The listing builds one solid part. Answer for the finished solid, in the listing's coordinates (mm). A direction names the side the tool comes from. Coordinates: 2 decimals unless noted, no trailing zeros. Order: outer loops, then holes, each group sorted by start corner. A loop starts at its lowest first (then second) coordinate and runs counter-clockwise, first axis right, second up. Notation, with made-up numbers: (-37, -8) -> (-11, -8) arc R22 ccw to (-11, 25) -> close; hole circle Ø11 at (20.5, -3.75). An arc over 180 degrees is marked (long way). Answer in a Markdown table with one row per item.
```python
from build123d import *

# Parameters (mm, degrees)
BOSS_EXTRUDE1_DEPTH          = 4
SKETCH3_R                    = 1.5
BOSS_EXTRUDE2_DEPTH          = 6
F_3_0_3_DIAMETER_HOLE1_D     = 3
F_3_0_3_DIAMETER_HOLE1_DEPTH = 10
FILLET2_R                    = 14.5
FILLET3_R                    = 2
CUT_EXTRUDE1_DEPTH           = 74.871510978
CUT_EXTRUDE1_DEPTH_BACK      = 7
SKETCH8_R                    = 46
SKETCH8_R_2                  = 9.814954576


with BuildPart() as part:
    # Sketch1 → Revolve1 (revolve)
    with BuildSketch(Plane(origin=(0, 0, 0), x_dir=(1, 0, 0), z_dir=(0, 1, 0))):
        Polygon((28, 45.5), (0, 45.5), (0, 16.5), (36, 16.5), (46, 26.5), (46, 40.5), align=None)
    revolve(axis=Axis((0, 0, -45.5), (0, 0, 1)))

    # Sketch2 → Boss-Extrude1 (add)
    with BuildSketch(Plane(origin=(0, 0, -45.5), x_dir=(-1, 0, 0), z_dir=(0, 0, -1))):
        Polygon((-9.814954576, 0), (-4.907477288, 8.5), (4.907477288, 8.5), (9.814954576, 0), (4.907477288, -8.5), (-4.907477288, -8.5), align=None)
    extrude(amount=BOSS_EXTRUDE1_DEPTH)

    # Sketch3 → Boss-Extrude2 (add)
    with BuildSketch(Plane.XY.offset(-16.5)):
        Circle(SKETCH3_R)
    extrude(amount=BOSS_EXTRUDE2_DEPTH)

    # Ø3.0 (3) Diameter Hole1
    with Locations(Plane.XY.offset(-16.5)):
        with Locations((-15.5, 0), (0, 15.5), (0, -15.5), (15.5, 0)):
            Hole(F_3_0_3_DIAMETER_HOLE1_D / 2, depth=F_3_0_3_DIAMETER_HOLE1_DEPTH)

    # Fillet2
    fillet2_edges = [part.edges().sort_by_distance(p)[0] for p in [
        (-36, 0, -16.5),
    ]]
    fillet(fillet2_edges, radius=FILLET2_R)

    # Fillet3
    fillet3_edges = [part.edges().sort_by_distance(p)[0] for p in [
        (-46, 0, -26.5),
    ]]
    fillet(fillet3_edges, radius=FILLET3_R)

    # Sketch8 → Cut-Extrude1 (cut, two sides: drawn at the far end of the back side and taken through both)
    with BuildSketch(Plane(origin=(0, 0, -45.5), x_dir=(-1, 0, 0), z_dir=(0, 0, -1)).offset(-CUT_EXTRUDE1_DEPTH_BACK)):
        Circle(SKETCH8_R)
        Circle(SKETCH8_R_2, mode=Mode.SUBTRACT)
    extrude(amount=CUT_EXTRUDE1_DEPTH + CUT_EXTRUDE1_DEPTH_BACK, mode=Mode.SUBTRACT)


solid = part.part
```
(1) A cutting plane is placed at B-B, the plane z = -15. Determine the outline of the cut face in (x, y).
Check values:
| item | result |
|---|---|
| outline | circle Ø3 at (0, 0) |
(2) For a pull along X with two mould halves and no side action, classify faces 1 (the flat face through (8, 5, -45.5)), 2 (the cylindrical face through (-1.5, 0.07, -13.54)), 3 (the flat face through (0, 16, -26.5)) as released by +X, released by -X, zero draft, split by the parting line, or undercut.
Check values:
| item | result |
|---|---|
| face 1 | zero draft |
| face 2 | split by the parting line |
| face 3 | undercut |
(3) A cutting plane is placed at A-A, the plane z = -47. Determine the outline of the cut face in (x, y), then the cut area to 3 significant figures.
Check values:
| item | result |
|---|---|
| outline | (-9.81, 0) -> (-4.91, -8.5) -> (4.91, -8.5) -> (9.81, 0) -> (4.91, 8.5) -> (-4.91, 8.5) -> close |
| area | 250 mm² |
(4) Find the intervals of material crossed by line 1 along X through (y, z) = (-15, -20); line 2 along Z through (x, y) = (20.5, 40.5); line 3 along Y through (x, z) = (15, -23.5), in increasing order. Write a range as from..to.
Check values:
| item | result |
|---|---|
| line 1 | -36.48..-1.41, 1.41..36.48 |
| line 2 | -38.5..-25.89 |
| line 3 | -40.3..-1.41, 1.41..40.3 |
(5) Which of the six approach directions +Z, -Z, +X, -X, +Y, -Y give full straight-line access (tool end or side, diameter ignored) to faces 4 (the flat face through (0, -8.5, -47)), 5 (the flat face through (7.396, 4.191, -47.472)), 6 (the cylindrical face through (7.234, 6.633, -41.951))?
Check values:
| item | result |
|---|---|
| face 4 | -Z, +X, -X, -Y |
| face 5 | -Z, +X, +Y |
| face 6 | -Z |
(6) Flat-ended cylindrical pins translate along their axes: pin 1 (2.5 mm diameter, centred on x = -15, y = -0.5, fed in from +Z); pin 2 (2.5 mm diameter, centred on x = 0, y = -15.5, fed in from +Z); pin 3 (1.5 mm diameter, centred on x = -8.5, y = 4.5, fed in from -Z); pin 4 (10 mm diameter, centred on y = -24.5, z = -45.5, fed in from +X). Find the tip coordinate at first contact, or state that the pin passes through.
Check values:
| item | result |
|---|---|
| pin 1 | z = -16.5 |
| pin 2 | z = -26.5 |
| pin 3 | z = -45.5 |
| pin 4 | through |
